Can you work these out from the model? Positions are in its coordinate system, mm. A direction names the side the tool comes from. Give positions to 0.01 mm unless a question says otherwise; leave off trailing zeros. Write each loop counter-clockwise with the first axis right and the second up, starting at its lowest first coordinate (ties: lowest second). Pieces come first, ordered by that corner, then holes.
```python
from build123d import *

# Parameters (mm, degrees)
SKETCH1_R           = 12.5349
BOSS_EXTRUDE1_DEPTH = 76.2
SKETCH2_R           = 4.7879
CUT_EXTRUDE1_DEPTH  = 76.2
SKETCH3_W           = 4.8514
SKETCH3_H           = 4.8514
BOSS_EXTRUDE2_DEPTH = 2.54
SKETCH4_R           = 7.4422
SKETCH4_R_2         = 4.7879
BOSS_EXTRUDE3_DEPTH = 3.81


with BuildPart() as part:
    # Sketch1 → Boss-Extrude1 (new body)
    with BuildSketch(Plane.XY):
        with Locations(Location((0, 0, 0), (0, 0, 180))):
            Circle(SKETCH1_R)
    extrude(amount=BOSS_EXTRUDE1_DEPTH)

    # Sketch2 → Cut-Extrude1 (cut)
    with BuildSketch(Plane(origin=(0, 10.16, 0), x_dir=(1, 0, 0), z_dir=(0, 1, 0))):
        with Locations(Location((0, -13.97, 0), (0, 0, 90))):
            Circle(SKETCH2_R)
    extrude(amount=CUT_EXTRUDE1_DEPTH, mode=Mode.SUBTRACT)

    # Sketch3 → Boss-Extrude2 (add)
    with BuildSketch(Plane(origin=(0, 10.16, 0), x_dir=(1, 0, 0), z_dir=(0, 1, 0))):
        with Locations((0, -13.97)):
            Rectangle(SKETCH3_W, SKETCH3_H)
    extrude(amount=BOSS_EXTRUDE2_DEPTH)

    # Sketch4 → Boss-Extrude3 (add)
    with BuildSketch(Plane(origin=(0, 10.16, 0), x_dir=(1, 0, 0), z_dir=(0, 1, 0))):
        with Locations(Location((0, -13.97, 0), (0, 0, 170.565483852))):
            Circle(SKETCH4_R)
        with Locations(Location((0, -13.97, 0), (0, 0, 90))):
            Circle(SKETCH4_R_2, mode=Mode.SUBTRACT)
    extrude(amount=BOSS_EXTRUDE3_DEPTH)


solid = part.part
```
1) Suppose I cut it at C-C on y = 6. Write out the boundary of the cut face in (x, z), plus the area to 3 significant figures.
Values follow:
outline: (-11.01, 0) - (11.01, 0) - (11.01, 76.2) - (-11.01, 76.2) - close
area: 1,680 mm2
2) For pin 1 Ø3 at (y, z) = (11.5, 14.5) entering from +X; pin 2 Ø2 at (y, z) = (2.5, 8) entering from -X; pin 3 Ø5 at (x, z) = (1, 29) entering from +Y, each with a flat end and sliding along its axis, tell me the tip position at first contact or that it passes through.
Values follow:
pin 1: stops at x = 7.56
pin 2: stops at x = -12.44
pin 3: stops at y = 12.53
3) Suppose I cut it at B-B on z = 13.97. Write out the boundary of the cut face in (x, y).
Values follow:
outline: (-7.44, 10.16) - (-7.34, 10.16) arc R12.53 ccw (long way) to (7.34, 10.16) - (7.44, 10.16) - (7.44, 13.97) - (4.79, 13.97) - (4.79, 10.16) - (2.43, 10.16) - (2.43, 12.7) - (-2.43, 12.7) - (-2.43, 10.16) - (-4.79, 10.16) - (-4.79, 13.97) - (-7.44, 13.97) - close
4) Please list where these lines run through material, in increasing order: L1, parallel to X at y = 12.65, z = 13.97; L2, parallel to X at y = 13.05, z = 13.97; L3, parallel to X at y = 0.5, z = 21.
Values follow:
L1: x = -7.44 to -4.79, -2.43 to 2.43, 4.79 to 7.44
L2: x = -7.44 to -4.79, 4.79 to 7.44
L3: x = -12.52 to 12.52
5) If we mould it in two halves opening along X, with no side actions, what happens to faces 1 (the face through (0, 11, 16.396)), 2 (the face through (0, 0, 76.2)), 3 (the face through (2.782, 12.462, 7.068))? For each: +X half, -X half, draft (parallel to the pull), parting line (faces both ways), or undercut.
Values follow:
face 1: undercut
face 2: draft
face 3: parting line
6) Suppose I cut it at A-A on x = 0. Write out the boundary of the cut face in (y, z).
Values follow:
outline: (-12.53, 0) - (12.53, 0) - (12.53, 6.53) - (13.97, 6.53) - (13.97, 9.18) - (10.16, 9.18) - (10.16, 11.54) - (12.7, 11.54) - (12.7, 16.4) - (10.16, 16.4) - (10.16, 18.76) - (13.97, 18.76) - (13.97, 21.41) - (12.53, 21.41) - (12.53, 76.2) - (-12.53, 76.2) - close
7) For faces 4 (the face through (1, 13.97, 9)), 5 (the face through (2.426, 11, 14)), which set-ups out of +Z, -Z, +X, -X, +Y, -Y let a thin tool reach every point of the face, with its end or its side?
Values follow:
face 4: +Z, -Z, +X, -X, +Y
face 5: +Y
8) Suppose I cut it at D-D on x = -6.5. Write out the boundary of the cut face in (y, z).
Values follow:
outline: (-10.72, 0) - (10.72, 0) - (10.72, 10.35) - (13.97, 10.35) - (13.97, 17.59) - (10.72, 17.59) - (10.72, 76.2) - (-10.72, 76.2) - close
